Part model, mm, in its own coordinate system. Face numbers are marked on the shaded views. A direction names the side the tool comes from. Round coordinates to 2 decimals unless told otherwise and drop trailing zeros. Loops run counter-clockwise (first coordinate to the right, second up) from the corner with the lowest first, then second, coordinate; pieces in that order, holes last.
(1) Flat gauge pins, fed straight in: pin 1 (3 mm diameter, centred on x = 5.66, y = 5.66, fed in from -Z); pin 2 (4.5 mm diameter, centred on x = -3.5, y = 9, fed in from +Z); pin 3 (5.5 mm diameter, centred on x = 5.66, y = 5.66, fed in from -Z); pin 4 (10 mm diameter, centred on x = -13, z = 23.5, fed in from -Y). Where does each tip first touch, or does it go through?
(2) Probe probe 1 along Z at (x, y) = (6.5, 8); probe 2 along Y at (x, z) = (-2, 8); probe 3 along Z at (x, y) = (-1.5, 15.75). List the from-to ranges inside material, lowest first.
(3) Cut at A-A on z = -6.5. Count the separate pieces of the cut face and the enclosed holes in it, then the cut area to 3 significant figures.
(4) Tool access for the marked faces 1, 2 and 3: list every direction of +Z, -Z, +X, -X, +Y, -Y with a clear straight run to the whole face (end or side of a thin tool).
(5) Cut at B-B on y = 9.5. List the corners of the cut face in (x, z) (3 decimals).
(6) Cut at C-C on x = 15.5. List the corners of the cut face in (y, z), then the cut area to 3 significant figures.
(7) Cut at D-D on y = 13.25. List the corners of the cut face in (x, z) (3 decimals).
from build123d import *

# Parameters (mm, degrees)
BOSS_EXTRUDE1_DEPTH = 38.1
SKETCH1_4_R         = 1.75
BOSS_EXTRUDE3_DEPTH = 7.5
SKETCH1_5_R         = 1.75
CUT_EXTRUDE1_DEPTH  = 1.75


with BuildPart() as part:
    # Sketch1 → Boss-Extrude1 (new body, symmetric)
    with BuildSketch(Plane.XY):
        Polygon((-7.875, 21.53615257), (7.875, 21.53615257), (33, 21.53615257), (33, 33.53615257), (-33, 33.53615257), (-33, 21.53615257), align=None)
    extrude(amount=BOSS_EXTRUDE1_DEPTH, both=True)

    # Sketch1_4 → Boss-Extrude3 (add, symmetric)
    with BuildSketch(Plane.XY):
        with BuildLine():
            ThreePointArc((-7.875, 7.68012858), (0, 11), (7.875, 7.68012858))
            Line((7.875, 7.68012858), (7.875, 21.53615257))
            Line((7.875, 21.53615257), (-7.875, 21.53615257))
            Line((-7.875, 21.53615257), (-7.875, 7.68012858))
        make_face()
        with BuildLine():
            ThreePointArc((1.951498019, 5.12615257), (3.835867687, 3.947771767), (6.019900654, 3.53615257))
            Line((6.019900654, 3.53615257), (6.125, 3.53615257))
            ThreePointArc((6.125, 3.53615257), (7.362436867, 4.048715703), (7.875, 5.28615257))
            Line((7.875, 5.28615257), (7.875, 7.68012858))
            ThreePointArc((7.875, 7.68012858), (0, 11), (-7.875, 7.68012858))
            Line((-7.875, 7.68012858), (-7.875, 5.28615257))
            ThreePointArc((-7.875, 5.28615257), (-7.362436867, 4.048715703), (-6.125, 3.53615257))
            Line((-6.125, 3.53615257), (-6.019900654, 3.53615257))
            ThreePointArc((-6.019900654, 3.53615257), (-3.835867687, 3.947771767), (-1.951498019, 5.12615257))
            Line((-1.951498019, 5.12615257), (-2.37323487, 4.737083337))
            ThreePointArc((-2.37323487, 4.737083337), (0, 5.664583337), (2.37323487, 4.737083337))
            Line((2.37323487, 4.737083337), (1.951498019, 5.12615257))
        make_face()
        with Locations((-5.656854249, 5.656854249)):
            Circle(SKETCH1_4_R, mode=Mode.SUBTRACT)
        with Locations((5.656854249, 5.656854249)):
            Circle(SKETCH1_4_R, mode=Mode.SUBTRACT)
    extrude(amount=BOSS_EXTRUDE3_DEPTH, both=True)

    # Sketch1_5 → Cut-Extrude1 (cut, symmetric)
    with BuildSketch(Plane.XY):
        with BuildLine():
            ThreePointArc((1.951498019, 5.12615257), (3.835867687, 3.947771767), (6.019900654, 3.53615257))
            Line((6.019900654, 3.53615257), (6.125, 3.53615257))
            ThreePointArc((6.125, 3.53615257), (7.362436867, 4.048715703), (7.875, 5.28615257))
            Line((7.875, 5.28615257), (7.875, 7.68012858))
            ThreePointArc((7.875, 7.68012858), (0, 11), (-7.875, 7.68012858))
            Line((-7.875, 7.68012858), (-7.875, 5.28615257))
            ThreePointArc((-7.875, 5.28615257), (-7.362436867, 4.048715703), (-6.125, 3.53615257))
            Line((-6.125, 3.53615257), (-6.019900654, 3.53615257))
            ThreePointArc((-6.019900654, 3.53615257), (-3.835867687, 3.947771767), (-1.951498019, 5.12615257))
            Line((-1.951498019, 5.12615257), (-2.37323487, 4.737083337))
            ThreePointArc((-2.37323487, 4.737083337), (0, 5.664583337), (2.37323487, 4.737083337))
            Line((2.37323487, 4.737083337), (1.951498019, 5.12615257))
        make_face()
        with Locations((-5.656854249, 5.656854249)):
            Circle(SKETCH1_5_R, mode=Mode.SUBTRACT)
        with Locations((5.656854249, 5.656854249)):
            Circle(SKETCH1_5_R, mode=Mode.SUBTRACT)
    extrude(amount=CUT_EXTRUDE1_DEPTH, both=True, mode=Mode.SUBTRACT)


solid = part.part
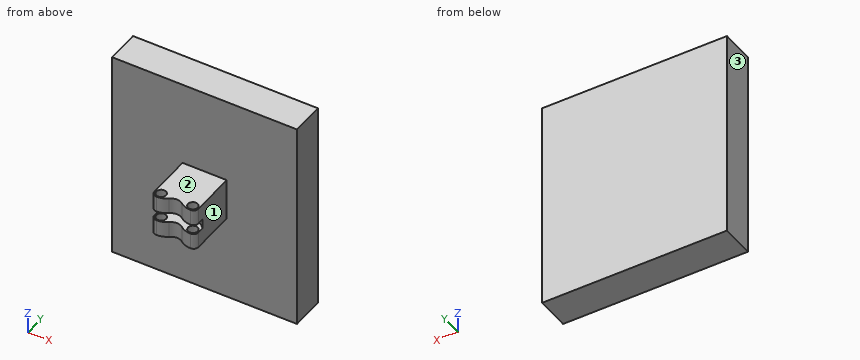
Final values:
1. pin 1: passes through
1. pin 2: stops at z = 7.5
1. pin 3: stops at z = -7.5
1. pin 4: stops at y = 21.54
2. probe 1: z = -7.5 to -1.75, 1.75 to 7.5
2. probe 2: y = 21.54 to 33.54
2. probe 3: z = -7.5 to 7.5
3. separate pieces: 1
3. enclosed holes: 2
3. area: 1,040 mm2
4. face 1: +Z, -Z, +X, -Y
4. face 2: +Z, +X, -X, -Y
4. face 3: +Z, -Z, -X, +Y, -Y
5. outline: (-7.875, -7.5) - (7.875, -7.5) - (7.875, 7.5) - (-7.875, 7.5) - close; hole (-5.545, -1.75) - (5.545, -1.75) - (5.545, 1.75) - (-5.545, 1.75) - close
6. outline: (21.54, -38.1) - (33.54, -38.1) - (33.54, 38.1) - (21.54, 38.1) - close
6. area: 914 mm2
7. outline: (-7.875, -7.5) - (7.875, -7.5) - (7.875, 7.5) - (-7.875, 7.5) - close
